The listing builds one solid part. Answer for the finished solid, in the listing's coordinates (mm). A direction names the side the tool comes from. Give positions to 0.01 mm unless a question says otherwise; leave off trailing zeros. Order: outer loops, then holes, each group sorted by start corner. A loop starts at its lowest first (then second) coordinate and runs counter-clockwise, first axis right, second up. Notation, with made-up numbers: (42.25, 68) - (79.25, 68) arc R23 ccw to (79.25, 91) - close; hole circle Ø11 at (49, 32). An arc over 180 degrees is marked (long way). Answer as a JSON object with one key per item and string values. Group by question number.
Q1. Consider line 1 (Y direction, x = -8.5, z = 4); line 2 (Z direction, x = 11.25, y = -7.5); line 3 (Y direction, x = 0.75, z = -35) (3 decimals). Determine where each line is inside the solid, lowest interval first.
Q2. Given pin 1 (10 mm diameter, centred on x = 7, y = 7.5, fed in from +Z); pin 2 (5.5 mm diameter, centred on y = -6.5, z = -39.5, fed in from -X); pin 3 (12 mm diameter, centred on x = 7.5, y = 5.5, fed in from +Z); pin 4 (6 mm diameter, centred on x = 4, y = 5.5, fed in from -Z), each flat-ended and moving along its own axis, determine where each tip first touches the part or whether it passes through.
Q3. A cutting plane is placed at C-C, the plane z = -13. Give the vertices of the cut face in (x, y), and give its area (3 significant figures).
Q4. For faces 1 (the face through (0, -1.225, -37)), 2 (the face through (11, -7, -25.95)), 3 (the face through (11.15, -7, -37)), determine the directions among +Z, -Z, +X, -X, +Y, -Y from which every point of the face is accessible in a straight line to the end or side of a thin tool.
Q5. A cutting plane is placed at A-A, the plane y = -12. Give the vertices of the cut face in (x, z), and give its area (3 significant figures).
Q6. A cutting plane is placed at B-B, the plane x = 0. Give the vertices of the cut face in (y, z) (3 decimals).
Q7. A cutting plane is placed at D-D, the plane x = 7. Give the vertices of the cut face in (y, z) (3 decimals), and give its area (3 significant figures).
from build123d import *

# Parameters (mm, degrees)
F0_W     = 19.9
F0_H     = 30.55
F1_DEPTH = 13.75
F3_DEPTH = 10.2
F5_W     = 24.6
F5_H     = 13.75
F6_DEPTH = 4.6
F7_W     = 22.3
F7_H     = 11.3
F8_DEPTH = 13.5


with BuildPart() as f1:
    # F0 (on Front) → F1 (new body)
    with BuildSketch(Plane.XZ):
        with BuildLine():
            ThreePointArc((9.95, 0), (0, 9.95), (-9.95, 0))
            Line((-9.95, 0), (9.95, 0))
        make_face()
        with Locations((0, -15.275)):
            Rectangle(F0_W, F0_H)
    extrude(amount=F1_DEPTH)

    # F2 (on face) → F3 (join)
    with BuildSketch(Plane(origin=(0, 0, 0), x_dir=(-1, 0, 0), z_dir=(0, 1, 0))):
        with BuildLine():
            ThreePointArc((1.095445115, -0.95), (1.3584725645, -0.5070032462), (1.45, 0))
            ThreePointArc((1.45, 0), (-0.5070032462, 1.3584725645), (-1.095445115, -0.95))
            Line((-1.095445115, -0.95), (1.095445115, -0.95))
        make_face()
        with BuildLine():
            Line((1.095445115, -0.95), (-1.095445115, -0.95))
            ThreePointArc((-1.095445115, -0.95), (0, -1.45), (1.095445115, -0.95))
        make_face()
    extrude(amount=F3_DEPTH)

    # F5 (on offset) → F6 (join)
    with BuildSketch(Plane(origin=(0, 0, -30.55), x_dir=(1, 0, 0), z_dir=(0, 0, -1))):
        with Locations((0, 6.875)):
            Rectangle(F5_W, F5_H)
    extrude(amount=-F6_DEPTH)

    # F7 (on offset) → F8 (join)
    with BuildSketch(Plane(origin=(0, 0, -30.55), x_dir=(1, 0, 0), z_dir=(0, 0, -1))):
        with Locations((0, 6.875)):
            Rectangle(F7_W, F7_H)
    extrude(amount=F8_DEPTH)


solid = f1.part
Reply:
{
 "1": {"line 1": "y = -13.75 to 0", "line 2": "z = -30.55 to -25.95", "line 3": "y = -12.525 to -1.225"},
 "2": {"pin 1": "passes through", "pin 2": "stops at x = -11.15", "pin 3": "stops at z = 8.54", "pin 4": "stops at z = -1.05"},
 "3": {"outline": "(-9.95, -13.75) - (9.95, -13.75) - (9.95, 0) - (-9.95, 0) - close", "area": "274 mm^2"},
 "4": {"face 1": "-Z, +X, -X, +Y", "face 2": "+Z, +X, +Y, -Y", "face 3": "-Z, +X, +Y, -Y"},
 "5": {"outline": "(-12.3, -30.55) - (-11.15, -30.55) - (-11.15, -44.05) - (11.15, -44.05) - (11.15, -30.55) - (12.3, -30.55) - (12.3, -25.95) - (9.95, -25.95) - (9.95, 0) arc R9.95 ccw to (-9.95, 0) - (-9.95, -25.95) - (-12.3, -25.95) - close", "area": "1,090 mm^2"},
 "6": {"outline": "(-13.75, -30.55) - (-12.525, -30.55) - (-12.525, -44.05) - (-1.225, -44.05) - (-1.225, -30.55) - (0, -30.55) - (0, -1.45) - (10.2, -1.45) - (10.2, 1.45) - (0, 1.45) - (0, 9.95) - (-13.75, 9.95) - close"},
 "7": {"outline": "(-13.75, -30.55) - (-12.525, -30.55) - (-12.525, -44.05) - (-1.225, -44.05) - (-1.225, -30.55) - (0, -30.55) - (0, 7.071) - (-13.75, 7.071) - close", "area": "670 mm^2"}
}
